from build123d import *

# Parameters (mm, degrees)
BASE_FLANGE1_DEPTH   = 3
EDGE_FLANGE1_START   = 13.5
EDGE_FLANGE1_DEPTH   = 24.4
EDGE_FLANGE1_START_2 = 113.5
EDGE_FLANGE1_2_DEPTH = 24.4
EDGE_FLANGE1_3_DEPTH = 1.5
EDGE_FLANGE1_START_3 = 36.4
EDGE_FLANGE1_4_DEPTH = 1.5
EDGE_FLANGE1_5_DEPTH = 1.5
EDGE_FLANGE1_START_4 = 136.4
EDGE_FLANGE1_6_DEPTH = 1.5
EDGE_FLANGE1_START_5 = 15
EDGE_FLANGE1_7_DEPTH = 21.4
EDGE_FLANGE1_START_6 = 115
EDGE_FLANGE1_8_DEPTH = 21.4
SKETCH12_R           = 3
CUT_EXTRUDE1_DEPTH   = 199.562861583
CUT_EXTRUDE2_DEPTH   = 201.701793714
FILLET1_R            = 5


# Read off the part's stored shape, not the designer's step: Edge-Flange1
# Sheet-metal steps are written as plain solids
with BuildPart() as part:
    # Sketch1 → Base-Flange1 (new body)
    with BuildSketch(Plane(origin=(0, 0, 0), x_dir=(0, 0, -1), z_dir=(1, 0, 0))):
        with BuildLine():
            Line((-89.400682252, 168.562214824), (-89.988204282, 151.737785176))
            ThreePointArc((-89.988204282, 151.737785176), (-90.094860642, 151.49823107), (-90.337991071, 151.4))
            Line((-90.337991071, 151.4), (-104.65, 151.4))
            Line((-104.65, 151.4), (-105, 151.4))
            Line((-105, 151.4), (-105, 151.05))
            Line((-105, 151.05), (-105, 136.592313107))
            Line((-105, 136.592313107), (-105, 136.4))
            Line((-105, 136.4), (-104.837845918, 136.296993093))
            ThreePointArc((-104.837845918, 136.296993093), (-50.024333792, 77.898717236), (-30.000377542, 0.349243281))
            Line((-30.000377542, 0.349243281), (-30, 0))
            Line((-30, 0), (-29.65037836, 0))
            Line((-29.65037836, 0), (-0.35, 0))
            Line((-0.35, 0), (0, 0))
            Line((0, 0), (0, 0.35))
            Line((0, 0.35), (0, 14.65))
            ThreePointArc((0, 14.65), (-0.102512627, 14.897487373), (-0.35, 15))
            Line((-0.35, 15), (-2, 15))
            Line((-2, 15), (-2, 15.7))
            Line((-2, 15.7), (-2, 35.7))
            Line((-2, 35.7), (-2, 36.4))
            Line((-2, 36.4), (-0.35, 36.4))
            ThreePointArc((-0.35, 36.4), (-0.102512627, 36.502512627), (0, 36.75))
            Line((0, 36.75), (0, 114.65))
            ThreePointArc((0, 114.65), (-0.102512627, 114.897487373), (-0.35, 115))
            Line((-0.35, 115), (-2, 115))
            Line((-2, 115), (-2, 115.7))
            Line((-2, 115.7), (-2, 135.7))
            Line((-2, 135.7), (-2, 136.4))
            Line((-2, 136.4), (-0.35, 136.4))
            ThreePointArc((-0.35, 136.4), (-0.102512627, 136.502512627), (0, 136.75))
            Line((0, 136.75), (0, 151.05))
            Line((0, 151.05), (0, 151.4))
            Line((0, 151.4), (-0.35, 151.4))
            Line((-0.35, 151.4), (-14.662008929, 151.4))
            ThreePointArc((-14.662008929, 151.4), (-14.905139358, 151.49823107), (-15.011795718, 151.737785176))
            Line((-15.011795718, 151.737785176), (-15.599317748, 168.562214824))
            ThreePointArc((-15.599317748, 168.562214824), (-15.705974108, 168.80176893), (-15.949104537, 168.9))
            Line((-15.949104537, 168.9), (-27.756435554, 168.9))
            ThreePointArc((-27.756435554, 168.9), (-27.969502054, 168.827673669), (-28.094509593, 168.640586666))
            Line((-28.094509593, 168.640586666), (-28.588074039, 166.798579077))
            ThreePointArc((-28.588074039, 166.798579077), (-28.597005701, 166.753676579), (-28.6, 166.707992411))
            Line((-28.6, 166.707992411), (-28.6, 153.25))
            ThreePointArc((-28.6, 153.25), (-28.702512627, 153.002512627), (-28.95, 152.9))
            Line((-28.95, 152.9), (-31.05, 152.9))
            ThreePointArc((-31.05, 152.9), (-31.297487373, 153.002512627), (-31.4, 153.25))
            Line((-31.4, 153.25), (-31.4, 166.707992411))
            ThreePointArc((-31.4, 166.707992411), (-31.402994299, 166.753676579), (-31.411925961, 166.798579077))
            Line((-31.411925961, 166.798579077), (-31.905490407, 168.640586666))
            ThreePointArc((-31.905490407, 168.640586666), (-32.030497946, 168.827673669), (-32.243564446, 168.9))
            Line((-32.243564446, 168.9), (-44.050895463, 168.9))
            ThreePointArc((-44.050895463, 168.9), (-44.294025892, 168.80176893), (-44.400682252, 168.562214824))
            Line((-44.400682252, 168.562214824), (-44.988204282, 151.737785176))
            ThreePointArc((-44.988204282, 151.737785176), (-45.094860642, 151.49823107), (-45.337991071, 151.4))
            Line((-45.337991071, 151.4), (-59.662008929, 151.4))
            ThreePointArc((-59.662008929, 151.4), (-59.905139358, 151.49823107), (-60.011795718, 151.737785176))
            Line((-60.011795718, 151.737785176), (-60.599317748, 168.562214824))
            ThreePointArc((-60.599317748, 168.562214824), (-60.705974108, 168.80176893), (-60.949104537, 168.9))
            Line((-60.949104537, 168.9), (-72.756435554, 168.9))
            ThreePointArc((-72.756435554, 168.9), (-72.969502054, 168.827673669), (-73.094509593, 168.640586666))
            Line((-73.094509593, 168.640586666), (-73.588074039, 166.798579077))
            ThreePointArc((-73.588074039, 166.798579077), (-73.597005701, 166.753676579), (-73.6, 166.707992411))
            Line((-73.6, 166.707992411), (-73.6, 153.25))
            ThreePointArc((-73.6, 153.25), (-73.702512627, 153.002512627), (-73.95, 152.9))
            Line((-73.95, 152.9), (-76.05, 152.9))
            ThreePointArc((-76.05, 152.9), (-76.297487373, 153.002512627), (-76.4, 153.25))
            Line((-76.4, 153.25), (-76.4, 166.707992411))
            ThreePointArc((-76.4, 166.707992411), (-76.402994299, 166.753676579), (-76.411925961, 166.798579077))
            Line((-76.411925961, 166.798579077), (-76.905490407, 168.640586666))
            ThreePointArc((-76.905490407, 168.640586666), (-77.030497946, 168.827673669), (-77.243564446, 168.9))
            Line((-77.243564446, 168.9), (-89.050895463, 168.9))
            ThreePointArc((-89.050895463, 168.9), (-89.294025892, 168.80176893), (-89.400682252, 168.562214824))
        make_face()
    extrude(amount=-BASE_FLANGE1_DEPTH)

    # Edge-Flange1 outline → Edge-Flange1 (cut)
    with BuildSketch(Plane(origin=(0, 0, 0), x_dir=(1, 0, 0), z_dir=(0, 1, 0)).offset(EDGE_FLANGE1_START)):
        with BuildLine():
            Line((0, -2), (-3, -2))
            Line((-3, -2), (-3, -3.755002002))
            ThreePointArc((-3, -3.755002002), (-0.788897449, -6.535898385), (0, -10))
            Line((0, -10), (0, -2))
        make_face()
    extrude(amount=EDGE_FLANGE1_DEPTH, mode=Mode.SUBTRACT)

    # Edge-Flange1 2 outline → Edge-Flange1 2 (cut)
    with BuildSketch(Plane(origin=(0, 0, 0), x_dir=(1, 0, 0), z_dir=(0, 1, 0)).offset(EDGE_FLANGE1_START_2)):
        with BuildLine():
            Line((0, -2), (-3, -2))
            Line((-3, -2), (-3, -3.755002002))
            ThreePointArc((-3, -3.755002002), (-0.788897449, -6.535898385), (0, -10))
            Line((0, -10), (0, -2))
        make_face()
    extrude(amount=EDGE_FLANGE1_2_DEPTH, mode=Mode.SUBTRACT)

    # Edge-Flange1 3 outline → Edge-Flange1 3 (cut)
    with BuildSketch(Plane(origin=(0, 0, 0), x_dir=(1, 0, 0), z_dir=(0, 1, 0)).offset(EDGE_FLANGE1_START)):
        with BuildLine():
            ThreePointArc((0, -10), (-0.788897449, -6.535898385), (-3, -3.755002002))
            Line((-3, -3.755002002), (-3, -11.5))
            Line((-3, -11.5), (0, -11.5))
            Line((0, -11.5), (0, -10))
        make_face()
    extrude(amount=EDGE_FLANGE1_3_DEPTH, mode=Mode.SUBTRACT)

    # Edge-Flange1 4 outline → Edge-Flange1 4 (cut)
    with BuildSketch(Plane(origin=(0, 0, 0), x_dir=(1, 0, 0), z_dir=(0, 1, 0)).offset(EDGE_FLANGE1_START_3)):
        with BuildLine():
            ThreePointArc((0, -10), (-0.788897449, -6.535898385), (-3, -3.755002002))
            Line((-3, -3.755002002), (-3, -11.5))
            Line((-3, -11.5), (0, -11.5))
            Line((0, -11.5), (0, -10))
        make_face()
    extrude(amount=EDGE_FLANGE1_4_DEPTH, mode=Mode.SUBTRACT)

    # Edge-Flange1 5 outline → Edge-Flange1 5 (cut)
    with BuildSketch(Plane(origin=(0, 0, 0), x_dir=(1, 0, 0), z_dir=(0, 1, 0)).offset(EDGE_FLANGE1_START_2)):
        with BuildLine():
            ThreePointArc((0, -10), (-0.788897449, -6.535898385), (-3, -3.755002002))
            Line((-3, -3.755002002), (-3, -11.5))
            Line((-3, -11.5), (0, -11.5))
            Line((0, -11.5), (0, -10))
        make_face()
    extrude(amount=EDGE_FLANGE1_5_DEPTH, mode=Mode.SUBTRACT)

    # Edge-Flange1 6 outline → Edge-Flange1 6 (cut)
    with BuildSketch(Plane(origin=(0, 0, 0), x_dir=(1, 0, 0), z_dir=(0, 1, 0)).offset(EDGE_FLANGE1_START_4)):
        with BuildLine():
            ThreePointArc((0, -10), (-0.788897449, -6.535898385), (-3, -3.755002002))
            Line((-3, -3.755002002), (-3, -11.5))
            Line((-3, -11.5), (0, -11.5))
            Line((0, -11.5), (0, -10))
        make_face()
    extrude(amount=EDGE_FLANGE1_6_DEPTH, mode=Mode.SUBTRACT)

    # Edge-Flange1 7 outline → Edge-Flange1 7 (add)
    with BuildSketch(Plane(origin=(0, 0, 0), x_dir=(1, 0, 0), z_dir=(0, 1, 0)).offset(EDGE_FLANGE1_START_5)):
        with BuildLine():
            Line((-3, -10), (-3, -3.755002002))
            ThreePointArc((-3, -3.755002002), (-5.350470229, -2.451490744), (-8, -2))
            Line((-8, -2), (-30, -2))
            Line((-30, -2), (-30, -5))
            Line((-30, -5), (-8, -5))
            ThreePointArc((-8, -5), (-4.464466094, -6.464466094), (-3, -10))
        make_face()
    extrude(amount=EDGE_FLANGE1_7_DEPTH)

    # Edge-Flange1 8 outline → Edge-Flange1 8 (add)
    with BuildSketch(Plane(origin=(0, 0, 0), x_dir=(1, 0, 0), z_dir=(0, 1, 0)).offset(EDGE_FLANGE1_START_6)):
        with BuildLine():
            Line((-3, -10), (-3, -3.755002002))
            ThreePointArc((-3, -3.755002002), (-5.350470229, -2.451490744), (-8, -2))
            Line((-8, -2), (-30, -2))
            Line((-30, -2), (-30, -5))
            Line((-30, -5), (-8, -5))
            ThreePointArc((-8, -5), (-4.464466094, -6.464466094), (-3, -10))
        make_face()
    extrude(amount=EDGE_FLANGE1_8_DEPTH)

    # Sketch12 → Cut-Extrude1 (cut, through all)
    with BuildSketch(Plane.XY.offset(5)):
        with Locations((-19, 125.7)):
            Circle(SKETCH12_R)
        with Locations((-19, 25.7)):
            Circle(SKETCH12_R)
    extrude(amount=-CUT_EXTRUDE1_DEPTH, mode=Mode.SUBTRACT)

    # Sketch14 → Cut-Extrude2 (cut, through all)
    with BuildSketch(Plane.ZY.offset(3)):
        with BuildLine():
            Line((2, 136.4), (0, 136.4))
            Line((0, 136.4), (0, 137.9))
            Line((0, 137.9), (0, 138.25))
            ThreePointArc((0, 138.25), (0.102512627, 138.002512627), (0.35, 137.9))
            Line((0.35, 137.9), (2, 137.9))
            Line((2, 137.9), (2, 136.4))
        make_face()
        with BuildLine():
            Line((2, 115), (0, 115))
            Line((0, 115), (0, 113.5))
            Line((0, 113.5), (0, 113.15))
            ThreePointArc((0, 113.15), (0.102512627, 113.397487373), (0.35, 113.5))
            Line((0.35, 113.5), (2, 113.5))
            Line((2, 113.5), (2, 115))
        make_face()
        with BuildLine():
            Line((2, 36.4), (0, 36.4))
            Line((0, 36.4), (0, 37.9))
            Line((0, 37.9), (0, 38.25))
            ThreePointArc((0, 38.25), (0.102512627, 38.002512627), (0.35, 37.9))
            Line((0.35, 37.9), (2, 37.9))
            Line((2, 37.9), (2, 36.4))
        make_face()
        with BuildLine():
            Line((2, 13.5), (2, 15))
            Line((2, 15), (0, 15))
            Line((0, 15), (0, 13.5))
            Line((0, 13.5), (0, 13.15))
            ThreePointArc((0, 13.15), (0.102512627, 13.397487373), (0.35, 13.5))
            Line((0.35, 13.5), (2, 13.5))
        make_face()
    extrude(amount=-CUT_EXTRUDE2_DEPTH, mode=Mode.SUBTRACT)

    # Fillet1
    fillet1_edges = [part.edges().sort_by_distance(p)[0] for p in [
        (-1.5, 136.4, 105),
        (-1.5, 151.4, 105),
        (-1.5, 151.4, 0),
        (-30, 115, 3.5),
        (-30, 136.4, 3.5),
        (-30, 36.4, 3.5),
        (-30, 15, 3.5),
        (-1.5, 0, 30),
        (-1.5, 0, 0),
    ]]
    fillet(fillet1_edges, radius=FILLET1_R)


solid = part.part
Here's how the part is built. I have some questions about the finished solid (model axes, mm). A direction names the side the tool comes from. Give positions to 0.01 mm unless a question says otherwise; leave off trailing zeros. Order: outer loops, then holes, each group sorted by start corner. A loop starts at its lowest first (then second) coordinate and runs counter-clockwise, first axis right, second up. Notation, with made-up numbers: (81, -6) -> (102, -6) arc R30 cw to (102, 20) -> close; hole circle Ø6 at (45.25, 34.5). An arc over 180 degrees is marked (long way). Use a Markdown table: item, result. Add a question column.
Item 1: For faces 5 (the face through (-1.52, 149.97, 1.5)), 6 (the face through (-16.7, 27.9, 5)), 7 (the face through (-12.7, 36.4, 4.6)), which set-ups out of +Z, -Z, +X, -X, +Y, -Y let a thin tool reach every point of the face, with its end or its side?
Item 2: Imagine slicing it at D-D on y = 25.7. Please give me the cut outline in (x, z) (3 decimals).
Item 3: Imagine slicing it at C-C on z = 19.5. Please give me the cut outline in (x, y).
Item 4: I need wall thicknesses on line 1 (Y direction, x = -19, z = 3); line 2 (Y direction, x = -14, z = 4); line 3 (Z direction, x = -27.5, y = 127). Which ranges of each line are inside material? Lowest first, please.
Item 5: Will these pins go through, and if not, where does the flat tip stop? pin 1 (4 mm diameter, centred on y = 67.5, z = 44, fed in from +X); pin 2 (17 mm diameter, centred on x = -22, y = 30, fed in from -Z); pin 3 (10.5 mm diameter, centred on x = -17, z = 8, fed in from -Y); pin 4 (2 mm diameter, centred on x = -25.5, y = 137.5, fed in from +Z).
Item 6: Imagine slicing it at B-B on y = 125.7. Please give me the cut outline in (x, z) (3 decimals).
Item 7: Imagine slicing it at A-A on x = -19. Please give me the cut outline in (y, z), plus the area to 3 significant figures.
Item 8: If we mould it in two halves opening along Y, with no side actions, what happens to faces 1 (the face through (-17, 123, 5)), 2 (the face through (-12.7, 136.4, 4.6)), 3 (the face through (-28.5, 34.97, 3.52)), 4 (the face through (-2, 2, 1))? For each: pulls with the +Y half, pulls with the -Y half, needs draft (parallel to the pull), parting line crosses it, or undercut.
Data:
| question | item | result |
|---|---|---|
| 1 | face 5 | -Z, +X, -X, +Y |
| 1 | face 6 | +Z, -X, +Y, -Y |
| 1 | face 7 | -Z, +X, -X |
| 2 | outline | (-30, 2) -> (-22, 2) -> (-22, 5) -> (-30, 5) -> close; (-16, 2) -> (-8, 2) arc R8 ccw to (0, 10) -> (0, 32.058) -> (-3, 32.058) -> (-3, 10) arc R5 cw to (-8, 5) -> (-16, 5) -> close |
| 3 | outline | (-3, 0) -> (0, 0) -> (0, 168.9) -> (-3, 168.9) -> close |
| 4 | line 1 | y = 15 to 22.7, 28.7 to 36.4, 115 to 122.7, 128.7 to 136.4 |
| 4 | line 2 | y = 15 to 36.4, 115 to 136.4 |
| 4 | line 3 | z = 2 to 5 |
| 5 | pin 1 | stops at x = 0 |
| 5 | pin 2 | stops at z = 2 |
| 5 | pin 3 | stops at y = 15 |
| 5 | pin 4 | passes through |
| 6 | outline | (-30, 2) -> (-22, 2) -> (-22, 5) -> (-30, 5) -> close; (-16, 2) -> (-8, 2) arc R8 ccw to (0, 10) -> (0, 90.081) -> (-3, 90.081) -> (-3, 10) arc R5 cw to (-8, 5) -> (-16, 5) -> close |
| 7 | outline | (15, 2) -> (22.7, 2) -> (22.7, 5) -> (15, 5) -> close; (28.7, 2) -> (36.4, 2) -> (36.4, 5) -> (28.7, 5) -> close; (115, 2) -> (122.7, 2) -> (122.7, 5) -> (115, 5) -> close; (128.7, 2) -> (136.4, 2) -> (136.4, 5) -> (128.7, 5) -> close |
| 7 | area | 92.4 mm² |
| 8 | face 1 | needs draft |
| 8 | face 2 | undercut |
| 8 | face 3 | undercut |
| 8 | face 4 | pulls with the -Y half |
